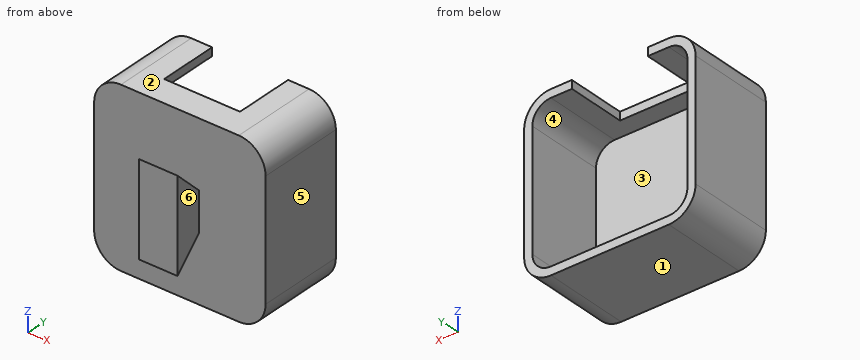
Autodesk Fusion 360 part; units mm, degrees
sketch "Sketch1" plane through (0, 0, 0) normal (0, 1, 0) x (1, 0, 0)
  line L0 (-15.85, 20.85) -> (15.85, 20.85)
  line L1 (20.85, 15.85) -> (20.85, -15.85)
  line L2 (15.85, -20.85) -> (-15.85, -20.85)
  line L3 (-20.85, -15.85) -> (-20.85, 15.85)
  line L4 (-20.85, 20.85) -> (20.85, -20.85) construction
  line L5 (20.85, 20.85) -> (-20.85, -20.85) construction
  arc A0 (-15.85, 20.85) -> (-20.85, 15.85) centre (-15.85, 15.85) ccw
  arc A1 (20.85, 15.85) -> (15.85, 20.85) centre (15.85, 15.85) ccw
  arc A2 (15.85, -20.85) -> (20.85, -15.85) centre (15.85, -15.85) ccw
  arc A3 (-20.85, -15.85) -> (-15.85, -20.85) centre (-15.85, -15.85) ccw
  arc A4 (23.05, 15.85) -> (15.85, 23.05) centre (15.85, 15.85) ccw
  line L6 (-15.85, 23.05) -> (15.85, 23.05)
  arc A5 (-15.85, 23.05) -> (-23.05, 15.85) centre (-15.85, 15.85) ccw
  line L7 (-23.05, -15.85) -> (-23.05, 15.85)
  arc A6 (-23.05, -15.85) -> (-15.85, -23.05) centre (-15.85, -15.85) ccw
  line L8 (15.85, -23.05) -> (-15.85, -23.05)
  arc A7 (15.85, -23.05) -> (23.05, -15.85) centre (15.85, -15.85) ccw
  line L9 (23.05, 15.85) -> (23.05, -15.85)
  dimension "d1" = 41.7
  dimension "d2" = 41.7
  dimension "d3" = 5
  dimension "d4" = -2.2
extrude "Extrude1" add sketch "Sketch1" along normal blind 2.2 contours L0 L1 L2 L3 A0 A1 A2 A3 | A4 L6 A5 L7 A6 L8 A7 L9
extrude "Extrude2" add sketch "Sketch1" along normal blind 23.4
sketch "Sketch2" plane through (0, 0, 23.05) normal (0, 0, 1) x (1, 0, 0)
  line L0 (-15.85, 0) -> (15.85, 0)
  line L1 (15.85, 0) -> (15.85, 23.4)
  line L2 (15.85, 23.4) -> (-15.85, 23.4)
  line L3 (-15.85, 23.4) -> (-15.85, 0)
  line L4 (10.2, 7.4) -> (-10.2, 7.4)
  line L5 (-10.2, 7.4) -> (-10.2, 23.4)
  line L6 (-10.2, 23.4) -> (10.2, 23.4)
  line L7 (10.2, 23.4) -> (10.2, 7.4)
  line L8 (-23.05, 0) -> (-23.05, 23.4)
  line L9 (23.05, 0) -> (23.05, 23.4)
  dimension "d9" = 7.4
  dimension "d10" = 20.4
  dimension "d11" = 16
  dimension "d13" = 12.85
  dimension "d14" = 12.85
extrude "Extrude3" cut sketch "Sketch2" against normal blind 2.2 contours L2 L4 L5 L6 L7
ref_plane "WorkPlane1" through (0, 11.7, 0) normal (1, 0, 0) x (0, 0, -1)
sketch "Sketch3" plane through (0, 0, 0) normal (1, 0, 0) x (0, 0, -1)
  line L0 (5.2, 0) -> (12.4125, -7.2125)
  line L1 (5.2, 0) -> (14.8, 0) construction
  line L2 (5.2, 0) -> (-5.2, 0)
  line L3 (-5.2, 0) -> (-12.4125, -7.2125)
  line L4 (12.4125, -7.2125) -> (-12.4125, -7.2125)
  point P0 (23.05, 0)
  point P1 (-23.05, 0)
  dimension "d18" = 10.2
  dimension "d19" = 45
  dimension "d20" = 45
  dimension "d21" = 10.2
  dimension "d22" = 10.4
  dimension "d23" = 17.85
  dimension "d24" = 17.85
extrude "Extrude4" add sketch "Sketch3" along normal mid plane 10.4
equation "d1 = 41.3 mm + 0.2 mm + 0.2 mm"
equation "d2 = 41.3 mm + 0.2 mm + 0.2 mm"
equation "d4 = -( 2 mm + 0.2 mm )"
equation "d5 = 2 mm + 0.2 mm"
equation "d7 = 2 mm + 0.2 mm + 21 mm + 0.2 mm"
equation "d9 = 2 mm + 0.2 mm + 5 mm + 0.2 mm"
equation "d10 = 20 mm + 0.2 mm + 0.2 mm"
equation "d11 = ( 2 mm + 0.2 mm + 21 mm + 0.2 mm ) - ( 2 mm + 0.2 mm + 5 mm + 0.2 mm )"
equation "d13 = Linear Dimension-5"
equation "d15 = -( 2 mm + 0.2 mm )"
equation "d17 = -( ( ( 41.3 + 0.2 + 0.2 + 2 + 0.2 + 2 + 0.2 ) / 2 ) * 1 mm )"
equation "d18 = 10 mm + 0.2 mm"
equation "d21 = 10 mm + 0.2 mm"
equation "d22 = 10 mm + 0.2 mm + 0.2 mm"
equation "d23 = ( ( ( 41.3 + 0.2 + 0.2 + 2 + 0.2 + 2 + 0.2 ) / 2 ) * 1 mm ) - ( 5 mm + 0.2 mm )"
equation "d25 = 5 mm + 0.2 mm"
The model under review builds one solid part; all positions refer to its coordinate system, in mm. Face numbers are marked on the shaded views. A direction names the side the tool comes from. Coordinates: 2 decimals unless noted, no trailing zeros. Loops run counter-clockwise (first coordinate to the right, second up) from the corner with the lowest first, then second, coordinate; pieces in that order, holes last. Notation, with made-up numbers: (72.5, 75) -> (117.5, 75) arc R20 cw to (117.5, 79) -> close; hole circle Ø5 at (9.25, 6). An arc over 180 degrees is marked (long way). Use a Markdown table: item, result. Add a question column.
1. Clearance check with flat-ended pins moving along their axes: pin 1 Ø1 at (y, z) = (17.5, 18) entering from -X; pin 2 Ø2 at (x, z) = (-6.5, -3.5) entering from +Y; pin 3 Ø3.5 at (y, z) = (-4, 1) entering from +X. State where each tip first meets the part, or that it passes through.
2. Add section B-B on x = -8. Write out the cut boundary in (y, z).
3. Add section C-C on y = 3.5. Write out the cut boundary in (x, z).
4. Add section D-D on z = -15. Write out the cut boundary in (x, y).
5. Machinability: for the marked faces 4, 5 and 6, which of the approach directions +Z, -Z, +X, -X, +Y, -Y give a long, thin tool a straight path to every point of the face, cutting with its end or side? Answer none if there is none.
6. Add section A-A on z = 11. Write out the cut boundary in (x, y), plus the area to 3 significant figures.
7. Draft analysis for pull direction Z (two halves, no side actions). For the marked faces 1, 2 and 3, state which applies: pulls with the +Z half, pulls with the -Z half, needs draft (parallel to the pull), parting line crosses it, or undercut.
8. To check wall thickness, follow line 1 (X direction, y = 12, z = 15); line 2 (Y direction, x = 0, z = -5). State the ranges of each line that lie inside material, in increasing order.
Returned:
| question | item | result |
|---|---|---|
| 1 | pin 1 | stops at x = -22.86 |
| 1 | pin 2 | stops at y = 2.2 |
| 1 | pin 3 | stops at x = 5.2 |
| 2 | outline | (0, -23.05) -> (23.4, -23.05) -> (23.4, -20.85) -> (2.2, -20.85) -> (2.2, 20.85) -> (7.4, 20.85) -> (7.4, 23.05) -> (0, 23.05) -> close |
| 3 | outline | (-23.05, -15.85) arc R7.2 ccw to (-15.85, -23.05) -> (15.85, -23.05) arc R7.2 ccw to (23.05, -15.85) -> (23.05, 15.85) arc R7.2 ccw to (15.85, 23.05) -> (-15.85, 23.05) arc R7.2 ccw to (-23.05, 15.85) -> close; hole (-20.85, -15.85) arc R5 ccw to (-15.85, -20.85) -> (15.85, -20.85) arc R5 ccw to (20.85, -15.85) -> (20.85, 15.85) arc R5 ccw to (15.85, 20.85) -> (-15.85, 20.85) arc R5 ccw to (-20.85, 15.85) -> close |
| 4 | outline | (-23.05, 0) -> (23.05, 0) -> (23.05, 23.4) -> (20.85, 23.4) -> (20.85, 2.2) -> (-20.85, 2.2) -> (-20.85, 23.4) -> (-23.05, 23.4) -> close |
| 5 | face 4 | +Y |
| 5 | face 5 | +Z, -Z, +X, +Y, -Y |
| 5 | face 6 | +Z, -Z, +X, -Y |
| 6 | outline | (-23.05, 0) -> (23.05, 0) -> (23.05, 23.4) -> (20.85, 23.4) -> (20.85, 2.2) -> (-20.85, 2.2) -> (-20.85, 23.4) -> (-23.05, 23.4) -> close; (-5.2, -7.21) -> (5.2, -7.21) -> (5.2, -5.8) -> (-5.2, -5.8) -> close |
| 6 | area | 209 mm² |
| 7 | face 1 | pulls with the -Z half |
| 7 | face 2 | pulls with the +Z half |
| 7 | face 3 | undercut |
| 8 | line 1 | x = -23.05 to -20.85, 20.85 to 23.05 |
| 8 | line 2 | y = -7.21 to 2.2 |
